from build123d import *

# Parameters (mm, degrees)
SKETCH1_W               = 16
SKETCH1_H               = 40
SKETCH1_R               = 2.5
BOSS_EXTRUDE1_DEPTH     = 3
BOSS_EXTRUDE3_START     = -3
SKETCH2_W               = 13
SKETCH2_H               = 3
SKETCH2_W_2             = 3
SKETCH2_H_2             = 34
BOSS_EXTRUDE3_DEPTH     = 93
CUT_EXTRUDE1_DEPTH      = 102.552941858
CUT_EXTRUDE1_DEPTH_BACK = 102.552941858
CUT_EXTRUDE2_START      = -1
SKETCH4_R               = 1.75
CUT_EXTRUDE2_DEPTH      = 102.493902258
SKETCH4_AGAIN_R         = 1.75
CUT_EXTRUDE3_DEPTH      = 103.493902258
FILLET1_R               = 0.7


with BuildPart() as part:
    # Sketch1 → Boss-Extrude1 (new body)
    with BuildSketch(Plane(origin=(0, 0, 0), x_dir=(1, 0, 0), z_dir=(0, 1, 0))):
        with Locations((0, 20)):
            Rectangle(SKETCH1_W, SKETCH1_H)
        with Locations(Location((0, 30, 0), (0, 0, 270))):
            Circle(SKETCH1_R, mode=Mode.SUBTRACT)
        with Locations(Location((0, 10, 0), (0, 0, 270))):
            Circle(SKETCH1_R, mode=Mode.SUBTRACT)
    extrude(amount=BOSS_EXTRUDE1_DEPTH)

    # Sketch2 → Boss-Extrude3 (add)
    with BuildSketch(Plane(origin=(0, 3, 0), x_dir=(1, 0, 0), z_dir=(0, 1, 0)).offset(BOSS_EXTRUDE3_START)):
        with Locations((1.5, 38.5)):
            Rectangle(SKETCH2_W, SKETCH2_H)
        with Locations((-6.5, 38.5)):
            Rectangle(SKETCH2_W_2, SKETCH2_H)
        with Locations((-6.5, 20)):
            Rectangle(SKETCH2_W_2, SKETCH2_H_2)
        with Locations((-6.5, 1.5)):
            Rectangle(SKETCH2_W_2, SKETCH2_H)
        with Locations((1.5, 1.5)):
            Rectangle(SKETCH2_W, SKETCH2_H)
    extrude(amount=BOSS_EXTRUDE3_DEPTH)

    # Sketch3 → Cut-Extrude1 (cut, two sides: drawn at the far end of the back side and taken through both)
    with BuildSketch(Plane(origin=(0, 0, -40), x_dir=(-1, 0, 0), z_dir=(0, 0, -1)).offset(-CUT_EXTRUDE1_DEPTH_BACK)):
        Polygon((-8, 6), (2, 93), (-8, 93), align=None)
    extrude(amount=CUT_EXTRUDE1_DEPTH + CUT_EXTRUDE1_DEPTH_BACK, mode=Mode.SUBTRACT)

    # Sketch4 → Cut-Extrude2 (cut, through all)
    # profile 1 of 2: a face of its own
    with BuildSketch(Plane.ZY.offset(8).offset(CUT_EXTRUDE2_START)):
        Polygon((-13.556624327, 76.5), (-12.113248654, 79), (-13.556624327, 81.5), (-16.443375673, 81.5), (-17.886751346, 79), (-16.443375673, 76.5), align=None)
        with Locations((-15, 79)):
            Circle(SKETCH4_R, mode=Mode.SUBTRACT)
    # profile 2 of 2: a face of its own
    with BuildSketch(Plane.ZY.offset(8).offset(CUT_EXTRUDE2_START)):
        Polygon((-23.556624327, 76.5), (-22.113248654, 79), (-23.556624327, 81.5), (-26.443375673, 81.5), (-27.886751346, 79), (-26.443375673, 76.5), align=None)
        with Locations((-25, 79)):
            Circle(SKETCH4_R, mode=Mode.SUBTRACT)
    extrude(amount=-CUT_EXTRUDE2_DEPTH, mode=Mode.SUBTRACT)

    # Sketch4 again → Cut-Extrude3 (cut, through all)
    with BuildSketch(Plane.ZY.offset(8)):
        with Locations((-25, 79)):
            Circle(SKETCH4_AGAIN_R)
        with Locations((-15, 79)):
            Circle(SKETCH4_AGAIN_R)
    extrude(amount=-CUT_EXTRUDE3_DEPTH, mode=Mode.SUBTRACT)

    # Fillet1
    fillet1_edges = [part.edges().sort_by_distance(p)[0] for p in [
        (3, 49.5, 0),
    ]]
    fillet(fillet1_edges, radius=FILLET1_R)
    fillet1_2_edges = [part.edges().sort_by_distance(p)[0] for p in [
        (3, 49.5, -3),
    ]]
    fillet(fillet1_2_edges, radius=FILLET1_R)
    fillet1_3_edges = [part.edges().sort_by_distance(p)[0] for p in [
        (3, 49.5, -40),
    ]]
    fillet(fillet1_3_edges, radius=FILLET1_R)
    fillet1_4_edges = [part.edges().sort_by_distance(p)[0] for p in [
        (3, 49.5, -37),
    ]]
    fillet(fillet1_4_edges, radius=FILLET1_R)


solid = part.part
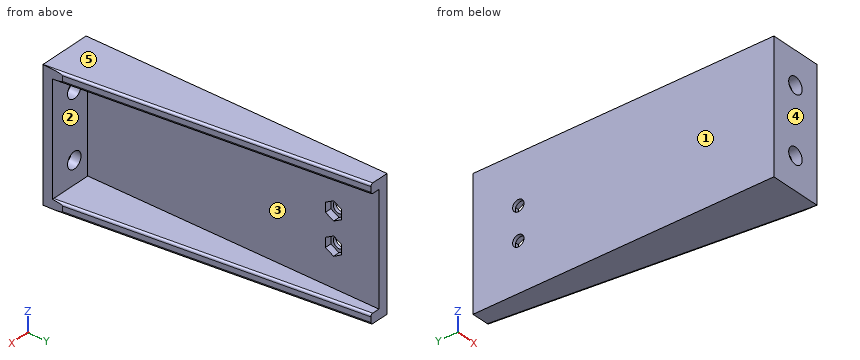
Can you work these out from the model? Positions are in its coordinate system, mm. Face numbers are marked on the shaded views. A direction names the side the tool comes from. Round coordinates to 2 decimals unless told otherwise and drop trailing zeros. Loops run counter-clockwise (first coordinate to the right, second up) from the corner with the lowest first, then second, coordinate; pieces in that order, holes last. Notation, with made-up numbers: (69.25, -33.5) - (77.25, -33.5) arc R20 ccw to (77.25, -0.5) - close; hole circle Ø6 at (64.5, 61). An arc over 180 degrees is marked (long way). Write item = value, one per line. Start each with the question number.
(1) If we section it at A-A (z = -31.5): Please give me the cut outline in (x, y).
(2) For P1, Ø4, axis at y = 42, z = -19.5, coming from the +X side; P2, Ø1.6, axis at x = -6, z = -14.5, coming from the -Y side; P3, Ø2, axis at x = 0.5, z = -8.5, coming from the +Y side, each with a flat end and sliding along its axis, tell me the tip position at first contact or that it passes through.
(3) If we section it at D-D (x = 0): Give the number of separate pieces and of enclosed holes in the cut face, and give its area (3 significant figures).
(4) If we mould it in two halves opening along Z, with no side actions, what happens to the marked faces 3, 4 and 5? For each: released by +Z, released by -Z, zero draft, split by the parting line, or undercut.
(5) For the marked faces 1 and 2, which set-ups out of +Z, -Z, +X, -X, +Y, -Y let a thin tool reach every point of the face, with its end or its side?
(6) If we section it at B-B (z = -25): Please give me the cut outline in (x, y).
(7) If I drill on probe 1 along Z at (x, y) = (-7.25, 79); probe 2 along Y at (x, z) = (-7.6, -25); probe 3 along Z at (x, y) = (-0.75, 15), over which ranges is the centre line in solid material (lowest first)? Write a range as [from, to].
(8) If we section it at C-C (z = -36): Please give me the cut outline in (x, y), and give its area (3 significant figures).
Ans:
q1.outline = (-8, 0) - (-2, 0) - (-2, 3) - (-5, 3) - (-5, 93) - (-8, 93) - close; (2, 0) - (8, 0) - (8, 3) - (2, 3) - close
q2.P1 = -5
q2.P2 = 0
q2.P3 = 3
q3.separate_pieces = 3
q3.enclosed_holes = 0
q3.area = 522 mm²
q4.face_3 = undercut
q4.face_4 = zero draft
q4.face_5 = released by +Z
q5.face_1 = +Z, -Z, -X, +Y, -Y
q5.face_2 = +X, +Y
q6.outline = (-8, 0) - (8, 0) - (8, 3) - (-5, 3) - (-5, 76.5) - (-7, 76.5) - (-7, 77.25) - (-8, 77.25) - close; (-8, 80.75) - (-7, 80.75) - (-7, 81.5) - (-5, 81.5) - (-5, 93) - (-8, 93) - close
q7.probe_1 = [-40, -26.75], [-23.25, -16.75], [-13.25, 0]
q7.probe_2 = [0, 77.25], [80.75, 93]
q7.probe_3 = [-40, -37], [-3, 0]
q8.outline = (-8, 0) - (8, 0) - (8, 3) - (-5, 3) - (-5, 93) - (-8, 93) - close
q8.area = 318 mm²
